```python
from build123d import *

# Parameters (mm, degrees)
BOSS_EXTRUDE1_DEPTH = 79
SKETCH2_W           = 38
SKETCH2_H           = 58
CUT_EXTRUDE1_DEPTH  = 79
SKETCH2_4_W         = 44
SKETCH2_4_H         = 64
SKETCH2_4_W_2       = 38
SKETCH2_4_H_2       = 58
BOSS_EXTRUDE2_DEPTH = 11.2
BOSS_EXTRUDE3_REACH = 88.426
BOSS_EXTRUDE4_REACH = 88.426
SKETCH2_9_W         = 44
SKETCH2_9_H         = 64
SKETCH2_9_W_2       = 38
SKETCH2_9_H_2       = 58
SKETCH3_W           = 4
SKETCH3_H           = 27.5
CUT_EXTRUDE2_DEPTH  = 11.2
SKETCH4_R           = 3.719736595
CUT_EXTRUDE3_DEPTH  = 11.2


with BuildPart() as part:
    # Sketch1 → Boss-Extrude1 (new body)
    with BuildSketch(Plane.XY):
        with BuildLine():
            Line((0, -15), (-16.986240344, -15))
            add(Edge.make_bspline(
                [(-25.5, -5.5), (-23.231190988, -6.092136591), (-20.857183856, -9.763256189), (-19.405733653, -14.032473401), (-16.986240344, -15)],
                knots=[0, 0, 0, 0, 0.466176326, 1, 1, 1, 1], degree=3))
            Line((-25.5, -5.5), (-32.550427966, -5.5))
            Line((-32.550427966, -5.5), (-32.550427966, -9))
            Line((-32.550427966, -9), (-27.122212975, -9))
            add(Edge.make_bspline(
                [(-27.122212975, -9), (-22.380611745, -10.95479786), (-23.823298098, -17.968578536), (-17.452262353, -18.5)],
                knots=[0, 0, 0, 0, 1, 1, 1, 1], degree=3))
            Line((-17.452262353, -18.5), (0, -18.5))
            Line((0, -18.5), (0, -15))
        make_face()
        with BuildLine():
            Line((16.986240344, -15), (0, -15))
            Line((0, -15), (0, -18.5))
            Line((0, -18.5), (17.452262353, -18.5))
            add(Edge.make_bspline(
                [(27.122212975, -9), (22.380611745, -10.95479786), (23.823298098, -17.968578536), (17.452262353, -18.5)],
                knots=[0, 0, 0, 0, 1, 1, 1, 1], degree=3))
            Line((27.122212975, -9), (32.550427966, -9))
            Line((32.550427966, -9), (32.550427966, -5.5))
            Line((32.550427966, -5.5), (25.5, -5.5))
            add(Edge.make_bspline(
                [(25.5, -5.5), (23.231190988, -6.092136591), (20.857183856, -9.763256189), (19.405733653, -14.032473401), (16.986240344, -15)],
                knots=[0, 0, 0, 0, 0.466176326, 1, 1, 1, 1], degree=3))
        make_face()
    extrude(amount=BOSS_EXTRUDE1_DEPTH)

    # Sketch2 → Cut-Extrude1 (cut)
    with BuildSketch(Plane.XZ.offset(18.5)):
        with Locations((0, 39.360513879)):
            Rectangle(SKETCH2_W, SKETCH2_H)
    extrude(amount=-CUT_EXTRUDE1_DEPTH, mode=Mode.SUBTRACT)

    # Sketch2_4 → Boss-Extrude2 (add)
    with BuildSketch(Plane.XZ.offset(18.5)):
        with Locations((0, 39.360513879)):
            Rectangle(SKETCH2_4_W, SKETCH2_4_H)
        with Locations((0, 39.360513879)):
            Rectangle(SKETCH2_4_W_2, SKETCH2_4_H_2, mode=Mode.SUBTRACT)
    extrude(amount=BOSS_EXTRUDE2_DEPTH)

    # Sketch2_8 → Boss-Extrude3 (add, up to next)
    with BuildSketch(Plane.XZ.offset(18.5), mode=Mode.PRIVATE) as boss_extrude3_sk1:
        Polygon((-19, 10.360513879), (-19, 68.360513879), (-17.452262353, 68.360513879), (-17.452262353, 71.360513879), (-22, 71.360513879), (-22, 7.360513879), (-17.452262353, 7.360513879), (-17.452262353, 10.360513879), align=None)
    boss_extrude3_tool1 = extrude(boss_extrude3_sk1.sketch, amount=-BOSS_EXTRUDE3_REACH, mode=Mode.PRIVATE) - part.part
    add(boss_extrude3_tool1.solids().sort_by_distance((-20.395094, -18.5, 39.360514))[0])

    # Sketch2_9 → Boss-Extrude4 (add, up to next)
    with BuildSketch(Plane.XZ.offset(18.5), mode=Mode.PRIVATE) as boss_extrude4_sk1:
        with Locations((0, 39.360513879)):
            Rectangle(SKETCH2_9_W, SKETCH2_9_H)
        with Locations((0, 39.360513879)):
            Rectangle(SKETCH2_9_W_2, SKETCH2_9_H_2, mode=Mode.SUBTRACT)
    boss_extrude4_tool1 = extrude(boss_extrude4_sk1.sketch, amount=-BOSS_EXTRUDE4_REACH, mode=Mode.PRIVATE) - part.part
    add(boss_extrude4_tool1.solids().sort_by_distance((21.22334, -18.5, 39.360514))[0])

    # Sketch3 → Cut-Extrude2 (cut)
    with BuildSketch(Plane.XZ.offset(9)):
        with Locations((29.122212975, 59.969493631)):
            Rectangle(SKETCH3_W, SKETCH3_H)
        with Locations((29.122212975, 19.030506369)):
            Rectangle(SKETCH3_W, SKETCH3_H)
    cut_extrude2 = extrude(amount=-CUT_EXTRUDE2_DEPTH, mode=Mode.SUBTRACT)

    # Mirror1: Cut-Extrude2 across plane
    add(cut_extrude2.mirror(Plane(origin=(0, 0, 0), x_dir=(0, 0, 1), z_dir=(1, 0, 0))), mode=Mode.SUBTRACT)

    # Sketch4 → Cut-Extrude3 (cut)
    with BuildSketch(Plane.ZY.offset(22)):
        with Locations((21.211295074, -29.7)):
            Circle(SKETCH4_R)
    extrude(amount=-CUT_EXTRUDE3_DEPTH, mode=Mode.SUBTRACT)


solid = part.part
```
CAD build for the part. Positions are in the model's coordinates, mm. A direction names the side the tool comes from. Round coordinates to 2 decimals unless told otherwise and drop trailing zeros. Order: outer loops, then holes, each group sorted by start corner. A loop starts at its lowest first (then second) coordinate and runs counter-clockwise, first axis right, second up.
Q1. Which spindle directions (+Z, -Z, +X, -X, +Y, -Y) get a long thin tool onto all of the face, cutting with end or side? Do faces 1 (the cylindrical face through (-20.52, -25.98, 21.29)), 2 (the flat face through (0, -18.5, 75)), 3 (the flat face through (22, -23, 39)), 4 (the flat face through (-19, -22, 39)). Say none if no direction does.
Q2. Slice it at C-C (y = -27.5). Write the cut outline in (x, z), and give its area (3 significant figures).
Q3. Slice it at A-A (x = -1.5). Write the cut outline in (y, z), and give its area (3 significant figures).
Q4. Drop flat-ended pins along their axis: pin 1 (6 mm diameter, centred on x = -8, z = 74, fed in from -Y); pin 2 (1.5 mm diameter, centred on x = -17.5, z = 18.5, fed in from +Y); pin 3 (5 mm diameter, centred on x = 18, y = -21.5, fed in from -Z); pin 4 (5 mm diameter, centred on y = -21.5, z = 39, fed in from +X). Give the stop position or say it passes through.
Q5. Wall check: L1, parallel to Z at x = -15, y = -17.75; L2, parallel to Z at x = -5.5, y = -26.5; L3, parallel to X at y = -19.5, z = 44.5. Give the ranges that are in metal, low to high.
Q6. Slice it at B-B (y = -23). Write the cut outline in (x, z), and give its area (3 significant figures).
Q7. Two-plate mould, pull along Z, no slides. Class faces 5 (the flat face through (0, -24, 7.361)), 6 (the flat face through (0, -18.5, 4)), 7 (the flat face through (27.122, -7, 19)), 8 (the flat face through (31.122, -7, 19)): pulls with the +Z half, pulls with the -Z half, needs draft (parallel to the pull), parting line crosses it, or undercut.
Q8. Slice it at D-D (z = 22.5). State how many separate pieces and enclosed holes the cut face has, and give its area (3 significant figures).
Results below:
1. face 1: -X, -Y
1. face 2: +Z, +X, -X, -Y
1. face 3: +Z, -Z, +X, -Y
1. face 4: +Y, -Y
2. outline: (-22, 7.36) - (22, 7.36) - (22, 71.36) - (-22, 71.36) - (-22, 24.21) - (-19, 24.21) - (-19, 68.36) - (19, 68.36) - (19, 10.36) - (-19, 10.36) - (-19, 18.21) - (-22, 18.21) - close
2. area: 594 mm2
3. outline: (-29.7, 7.36) - (-18.5, 7.36) - (-18.5, 0) - (-15, 0) - (-15, 10.36) - (-29.7, 10.36) - close; (-29.7, 68.36) - (-15, 68.36) - (-15, 79) - (-18.5, 79) - (-18.5, 71.36) - (-29.7, 71.36) - close
3. area: 141 mm2
4. pin 1: stops at y = -29.7
4. pin 2: passes through
4. pin 3: stops at z = 7.36
4. pin 4: stops at x = 22
5. L1: z = 0 to 10.36, 68.36 to 79
5. L2: z = 7.36 to 10.36, 68.36 to 71.36
5. L3: x = -22 to -19, 19 to 22
6. outline: (-22, 7.36) - (22, 7.36) - (22, 71.36) - (-22, 71.36) - close; hole (-19, 10.36) - (19, 10.36) - (19, 68.36) - (-19, 68.36) - close
6. area: 612 mm2
7. face 5: pulls with the -Z half
7. face 6: needs draft
7. face 7: undercut
7. face 8: undercut
8. separate pieces: 4
8. enclosed holes: 0
8. area: 168 mm2
